```python
from build123d import *

# Parameters (mm, degrees)
F1_DEPTH = 150
F4_DEPTH = 14.6
F7_DEPTH = 25


with BuildPart() as f1:
    # F0 (on Top) → F1 (new body)
    with BuildSketch(Plane.XY):
        with BuildLine():
            ThreePointArc((-20.1233408974, -5.9455809682), (-31.1901518255, -3.7500670345), (-27.5583376919, 6.9319043027))
            ThreePointArc((-27.5583376919, 6.9319043027), (-24.6952207253, 28.5156271448), (-7.4348638898, 41.787198732))
            ThreePointArc((-7.4348638898, 41.787198732), (0, 50.2735044354), (7.4348638898, 41.787198732))
            ThreePointArc((7.4348638898, 41.787198732), (24.6952207253, 28.5156271448), (27.5583376919, 6.9319043027))
            ThreePointArc((27.5583376919, 6.9319043027), (31.1901518255, -3.7500670345), (20.1233408974, -5.9455809682))
            Line((20.1233408974, -5.9455809682), (18.9042318034, -7.5310692264))
            ThreePointArc((18.9042318034, -7.5310692264), (32.4530777326, -5.4829034184), (29.8611497399, 7.9725088187))
            ThreePointArc((29.8611497399, 7.9725088187), (26.4272766932, 29.5156182068), (9.4874750724, 43.2611690236))
            ThreePointArc((9.4874750724, 43.2611690236), (0, 52.2735044354), (-9.4874750724, 43.2611690236))
            ThreePointArc((-9.4874750724, 43.2611690236), (-26.4272766932, 29.5156182068), (-29.8611497399, 7.9725088187))
            ThreePointArc((-29.8611497399, 7.9725088187), (-32.4530777326, -5.4829034184), (-18.9042318034, -7.5310692264))
            Line((-18.9042318034, -7.5310692264), (-20.1233408974, -5.9455809682))
        make_face()
    extrude(amount=F1_DEPTH)

    # F3 (on 3pt) → F4 (cut)
    with BuildSketch(Plane(origin=(25.8481727674, 14.9232716588, 0), x_dir=(0.499995531, -0.8660279839, 0), z_dir=(-0.8660279839, -0.499995531, 0))):
        with BuildLine():
            Line((-7.3478311295, 20), (-7.3478311295, 130))
            ThreePointArc((-7.3478311295, 130), (-8.8122972235, 133.5355339059), (-12.3478311295, 135))
            ThreePointArc((-12.3478311295, 135), (-15.8833650354, 133.5355339059), (-17.3478311295, 130))
            Line((-17.3478311295, 130), (-17.3478311295, 20))
            ThreePointArc((-17.3478311295, 20), (-15.8833650354, 16.4644660941), (-12.3478311295, 15))
            ThreePointArc((-12.3478311295, 15), (-8.8122972235, 16.4644660941), (-7.3478311295, 20))
        make_face()
    extrude(amount=-F4_DEPTH, mode=Mode.SUBTRACT)

    # F6 (on 3pt) → F7 (cut)
    with BuildSketch(Plane(origin=(-25.8481727674, 14.9232716588, 0), x_dir=(-0.499995531, -0.8660279839, 0), z_dir=(-0.8660279839, 0.499995531, 0))):
        with BuildLine():
            ThreePointArc((-12.3478310445, 135), (-15.8833649505, 133.5355339059), (-17.3478310445, 130))
            Line((-17.3478310445, 130), (-17.3478310445, 20))
            ThreePointArc((-17.3478310445, 20), (-15.8833649505, 16.4644660941), (-12.3478310445, 15))
            ThreePointArc((-12.3478310445, 15), (-8.8122971386, 16.4644660941), (-7.3478310445, 20))
            Line((-7.3478310445, 20), (-7.3478310445, 130))
            ThreePointArc((-7.3478310445, 130), (-8.8122971386, 133.5355339059), (-12.3478310445, 135))
        make_face()
    extrude(amount=F7_DEPTH, mode=Mode.SUBTRACT)


solid = f1.part
```
Can you work these out from the model? Positions are in its coordinate system, mm. A direction names the side the tool comes from. Give positions to 0.01 mm unless a question says otherwise; leave off trailing zeros. Order: outer loops, then holes, each group sorted by start corner. A loop starts at its lowest first (then second) coordinate and runs counter-clockwise, first axis right, second up. Notation, with made-up numbers: (46.25, 23.5) - (60.25, 23.5) arc R22 cw to (60.25, 34.5) - close; hole circle Ø7 at (72, 36.5). An arc over 180 degrees is marked (long way). Use a Markdown table: item, result. Add a question column.
Q1. I'm going to push flat-ended pins straight in: pin 1 (5 mm diameter, centred on y = -3.5, z = 116.5, fed in from +X); pin 2 (10 mm diameter, centred on y = 45.5, z = 40.5, fed in from +X); pin 3 (8 mm diameter, centred on x = -2.5, z = 33.5, fed in from +Y); pin 4 (2 mm diameter, centred on x = 11.5, z = 59, fed in from -Y). Where does each tip first touch, or does it pass through?
Q2. Please list where these lines run through material, in increasing order: line 1 along X through (y, z) = (0, 47.5) (3 decimals); line 2 along X through (y, z) = (43.5, 119); line 3 along Y through (x, z) = (-24, 84).
Q3. If we section it at C-C on y = 40: Write out the boundary of the cut face in (x, z).
Q4. If we section it at A-A on y = 0: Write out the boundary of the cut face in (x, z) (3 decimals), plus the area to 3 significant figures.
Q5. If we section it at D-D on z = 140.5: Write out the boundary of the cut face in (x, y) (1 decimal).
Q6. On a 3-axis mill with a long thin cutter (end or side, diameter ignored), from which of +Z, -Z, +X, -X, +Y, -Y can I reach the whole of each face in a straight line? I mean faces 1 (the flat face through (-8, 42, 0)), 2 (the cylindrical face through (-26.897, 23.728, 73.95)). Say none if no direction works.
Q7. If we section it at B-B on z = 17.5: Write out the boundary of the cut face in (x, y) (1 decimal).
Q8. If we mould it in two halves opening along Y, with no side actions, what happens to faces 3 (the cylindrical face through (0.2, 52.27, 73.95)), 4 (the flat face through (-8, 42, 150)), 5 (the cylindrical face through (31.28, -3.59, 73.95))? For each: released by +Y, released by -Y, zero draft, split by the parting line, or undercut.
Answers follow:
| question | item | result |
|---|---|---|
| 1 | pin 1 | stops at x = 34.14 |
| 1 | pin 2 | stops at x = 15.57 |
| 1 | pin 3 | stops at y = 52.27 |
| 1 | pin 4 | stops at y = 39.89 |
| 2 | line 1 | x = -34.195 to -32.195, 32.195 to 34.195 |
| 2 | line 2 | x = -9.47 to -7.46, 7.46 to 9.47 |
| 2 | line 3 | y = -9.47 to -7.47 |
| 3 | outline | (-16.39, 0) - (-12.27, 0) - (-12.27, 150) - (-16.39, 150) - close; (12.27, 0) - (16.39, 0) - (16.39, 150) - (12.27, 150) - close |
| 4 | outline | (-34.195, 0) - (-32.195, 0) - (-32.195, 150) - (-34.195, 150) - close; (32.195, 0) - (34.195, 0) - (34.195, 150) - (32.195, 150) - close |
| 4 | area | 600 mm^2 |
| 5 | outline | (-29.9, 8) arc R9.5 ccw (long way) to (-18.9, -7.5) - (-20.1, -5.9) arc R7.5 cw (long way) to (-27.6, 6.9) arc R28.5 cw to (-7.4, 41.8) arc R7.5 cw (long way) to (7.4, 41.8) arc R28.5 cw to (27.6, 6.9) arc R7.5 cw (long way) to (20.1, -5.9) - (18.9, -7.5) arc R9.5 ccw (long way) to (29.9, 8) arc R30.5 ccw to (9.5, 43.3) arc R9.5 ccw to (-9.5, 43.3) arc R30.5 ccw to start |
| 6 | face 1 | -Z, +X, -X, +Y, -Y |
| 6 | face 2 | +Z, -Z |
| 7 | outline | (-29.9, 8) arc R9.5 ccw (long way) to (-18.9, -7.5) - (-20.1, -5.9) arc R7.5 cw (long way) to (-27.6, 6.9) arc R28.5 cw to (-26.6, 24.6) - (-28.3, 25.6) arc R30.5 ccw to start; (-24, 33.1) - (-22.2, 32.1) arc R28.5 cw to (-7.4, 41.8) arc R7.5 cw (long way) to (7.4, 41.8) arc R28.5 cw to (22.2, 32.1) - (24, 33.1) arc R30.5 ccw to (9.5, 43.3) arc R9.5 ccw to (-9.5, 43.3) arc R30.5 ccw to start; (18.9, -7.5) arc R9.5 ccw (long way) to (29.9, 8) arc R30.5 ccw to (28.3, 25.6) - (26.6, 24.6) arc R28.5 cw to (27.6, 6.9) arc R7.5 cw (long way) to (20.1, -5.9) - close |
| 8 | face 3 | released by +Y |
| 8 | face 4 | zero draft |
| 8 | face 5 | undercut |
